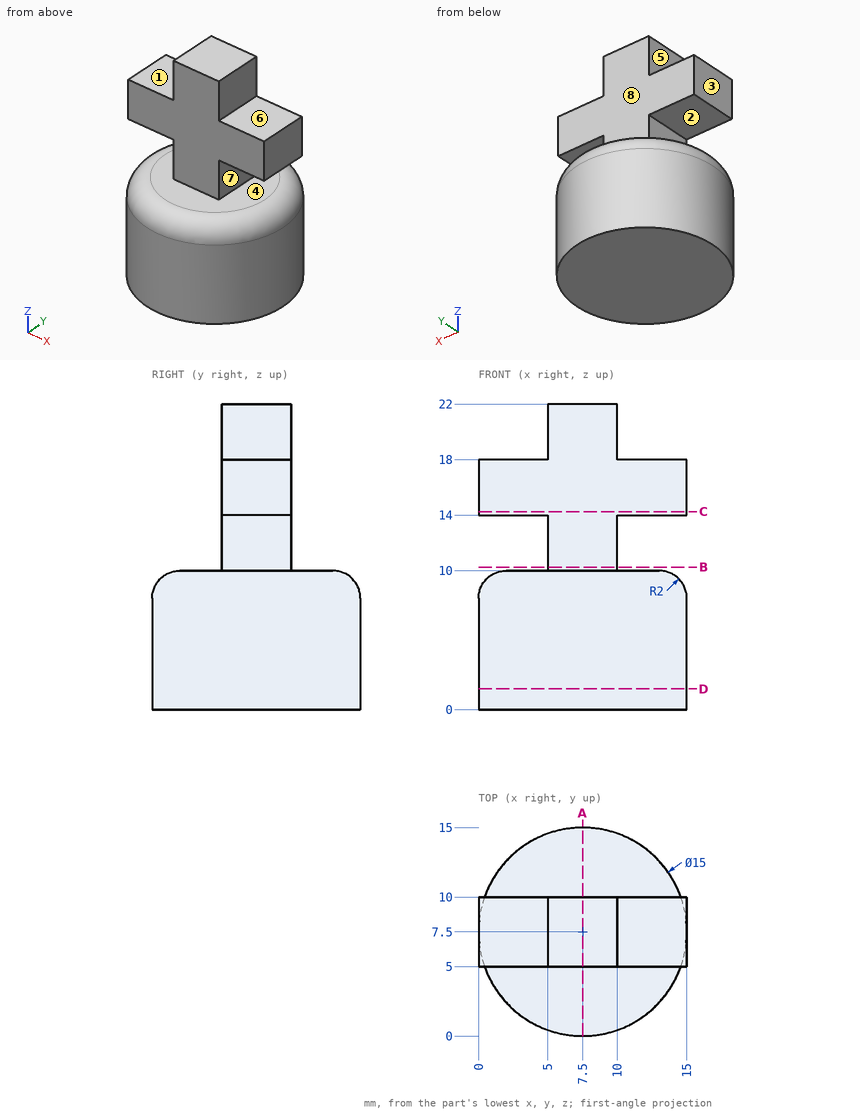
Can you work these out from the drawing? Everything is in mm from the part's minimum corner. A direction names the side the tool comes from. Round coordinates to 2 decimals unless told otherwise and drop trailing zeros. Loops run counter-clockwise (first coordinate to the right, second up) from the corner with the lowest first, then second, coordinate; pieces in that order, holes last. Notation, with made-up numbers: (86, 6.25) - (105, 6.25) arc R25 cw to (105, 18.25) - close; hole circle Ø5 at (5.25, -10). An arc over 180 degrees is marked (long way). One line per question, with ' | ' between items. Start each with the question number.
Q1. I want a section at A-A (x = 7.5). Write out the boundary of the cut face in (y, z).
Q2. We'd pull the mould along Z, two halves only. Please class the marked faces 1, 2, 3 and 4: +Z half, -Z half, draft (parallel to the pull), parting line (faces both ways), or undercut.
Q3. Will these pins go through, and if not, where does the flat tip stop? pin 1 (4.5 mm diameter, centred on y = 7.5, z = 20, fed in from -X); pin 2 (4 mm diameter, centred on x = 13.5, y = 8.5, fed in from +Z); pin 3 (1 mm diameter, centred on y = 4.5, z = 5, fed in from -X); pin 4 (8 mm diameter, centred on x = 1.5, z = 9, fed in from +Y).
Q4. I want a section at C-C (z = 14.25). Write out the boundary of the cut face in (x, y), then the cut area to 3 significant figures.
Q5. For the marked faces 5, 6, 7 and 8, which set-ups out of +Z, -Z, +X, -X, +Y, -Y let a thin tool reach every point of the face, with its end or its side?
Q6. I want a section at B-B (z = 10.25). Write out the boundary of the cut face in (x, y), then the cut area to 3 significant figures.
Q7. I want a section at D-D (z = 1.5). Write out the boundary of the cut face in (x, y).
Q8. Please list where these lines run through material, in increasing order: line 1 (Z direction, x = 2.75, y = 8.75); line 2 (Y direction, x = 5.75, z = 14); line 3 (Z direction, x = 7.5, y = 12.25). Write a range as [from, to].
Response values:
1) outline: (0, 0) - (15, 0) - (15, 8) arc R2 ccw to (13, 10) - (10, 10) - (10, 22) - (5, 22) - (5, 10) - (2, 10) arc R2 ccw to (0, 8) - close
2) face 1: +Z half | face 2: undercut | face 3: draft | face 4: undercut
3) pin 1: stops at x = 0 | pin 2: stops at z = 18 | pin 3: stops at x = 0.43 | pin 4: stops at y = 14.7
4) outline: (0, 5) - (15, 5) - (15, 10) - (0, 10) - close | area: 75.0 mm²
5) face 5: +Z, -X, +Y, -Y | face 6: +Z, +X, +Y, -Y | face 7: +X, +Y, -Y | face 8: +Z, +X, -X, +Y
6) outline: (5, 5) - (10, 5) - (10, 10) - (5, 10) - close | area: 25.0 mm²
7) outline: circle Ø15 at (7.5, 7.5)
8) line 1: z = [0, 10], [14, 18] | line 2: y = [5, 10] | line 3: z = [0, 10]
